Could you check a few things on this model? Use its own coordinates, in mm. A direction names the side the tool comes from. Give positions to 0.01 mm unless a question says otherwise; leave off trailing zeros. Write each loop counter-clockwise with the first axis right and the second up, starting at its lowest first coordinate (ties: lowest second). Pieces come first, ordered by that corner, then holes. Notation, with made-up numbers: M 28,-10 L 68,-10 A18 ccw 68,10 Z; hole C -29.75,55 d9. An arc over 180 degrees is marked long. One line per item, written item: value.
```python
from build123d import *

# Parameters (mm, degrees)
PAD_DEPTH            = 10
PAD002_DEPTH         = 29.635
POCKET_DEPTH         = 0.001
POCKET_DEPTH_BACK    = -14.001
SKETCH004_W          = 82.61631
SKETCH004_H          = 35.698411
SKETCH004_W_2        = 63.407177
SKETCH004_H_2        = 4.929781
POCKET001_DEPTH      = 17.005409
POCKET001_DEPTH_BACK = -17.005409


with BuildPart() as part:
    # Sketch → Pad (new body)
    with BuildSketch(Plane.XY):
        Polygon((19.635, 0), (9.8175, 17.004409), (-9.8175, 17.004409), (-19.635, 0), (-9.8175, -17.004409), (9.8175, -17.004409), align=None)
        Polygon((13.635, 0), (6.8175, 11.808256), (-6.8175, 11.808256), (-13.635, 0), (-6.8175, -11.808256), (6.8175, -11.808256), align=None, mode=Mode.SUBTRACT)
    extrude(amount=PAD_DEPTH)

    # Sketch002 → Pad002 (join, symmetric)
    with BuildSketch(Plane.YZ):
        with BuildLine():
            ThreePointArc((4, 10), (0, 14), (-4, 10))
            Line((-4, 10), (-4, 0))
            Line((-4, 0), (4, 0))
            Line((4, 0), (4, 10))
        make_face()
    extrude(amount=PAD002_DEPTH, both=True)

    # Sketch003 → Pocket (cut, two sides)
    with BuildSketch(Plane.XY) as pocket_sk:
        Polygon((13.635, 0), (6.8175, 11.808256), (-6.8175, 11.808256), (-13.635, 0), (-6.8175, -11.808256), (6.8175, -11.808256), align=None)
    extrude(amount=-POCKET_DEPTH, mode=Mode.SUBTRACT)
    extrude(pocket_sk.sketch, amount=-POCKET_DEPTH_BACK, mode=Mode.SUBTRACT)

    # Sketch004 → Pocket001 (cut, two sides)
    with BuildSketch(Plane.XZ) as pocket001_sk:
        with Locations((0.841957, 8.089457)):
            Rectangle(SKETCH004_W, SKETCH004_H)
        with Locations((0.246989, 0.581458)):
            Rectangle(SKETCH004_W_2, SKETCH004_H_2, mode=Mode.SUBTRACT)
    extrude(amount=-POCKET001_DEPTH, mode=Mode.SUBTRACT)
    extrude(pocket001_sk.sketch, amount=-POCKET001_DEPTH_BACK, mode=Mode.SUBTRACT)


solid = part.part
```
1) If we section it at A-A, the plane x = 1: Write out the boundary of the cut face in (y, z).
Outcome:
outline: M -17,0 L -11.81,0 L -11.81,3.05 L -17,3.05 Z; M 11.81,0 L 17,0 L 17,3.05 L 11.81,3.05 Z
2) We'd pull the mould along X, two halves only. Please class faces 1 (the face through (0, -17.004, 2)), 2 (the face through (-29.635, 0, 2)), 3 (the face through (13.624, 10.411, 1.502)), 4 (the face through (10.274, 5.821, 1.502)): pulls with the +X half, pulls with the -X half, needs draft (parallel to the pull), parting line crosses it, or undercut.
Outcome:
face 1: needs draft
face 2: pulls with the -X half
face 3: pulls with the +X half
face 4: undercut
3) On a 3-axis mill with a long thin cutter (end or side, diameter ignored), from which of +Z, -Z, +X, -X, +Y, -Y can I reach the whole of each face in a straight line? I mean faces 5 (the face through (-23, 4, 2)), 6 (the face through (24, 4, 2)), 7 (the face through (-23, -4, 2)), 8 (the face through (-10.274, -5.821, 1.502)), 9 (the face through (24, -4, 2)). Say none if no direction works.
Outcome:
face 5: +Z, -Z, -X, +Y
face 6: +Z, -Z, +X, +Y
face 7: +Z, -Z, -X, -Y
face 8: +Z, -Z
face 9: +Z, -Z, +X, -Y
4) If we section it at D-D, the plane x = 18: Write out the boundary of the cut face in (y, z).
Outcome:
outline: M -4,0 L 4,0 L 4,3.05 L -4,3.05 Z
5) I'm going to push flat-ended pins straight in: pin 1 (1.5 mm diameter, centred on x = -25, z = 1, fed in from -Y); pin 2 (1 mm diameter, centred on y = -5.5, z = 2.5, fed in from +X). Where does each tip first touch, or does it pass through?
Outcome:
pin 1: stops at y = -4
pin 2: stops at x = 16.75
6) Please list where these lines run through material, in increasing order: L1, parallel to Y at x = 3.5, z = 2.5; L2, parallel to X at y = 0, z = 0.8 (3 decimals); L3, parallel to Y at x = -19.5, z = 2.1. Write a range as from..to.
Outcome:
L1: y = -17..-11.81, 11.81..17
L2: x = -29.635..-13.635, 13.635..29.635
L3: y = -4..4
7) If we section it at C-C, the plane z = 2.4: Write out the boundary of the cut face in (x, y) (1 decimal), then the cut area to 3 significant figures.
Outcome:
outline: M -29.6,-4 L -17.3,-4 L -9.8,-17 L 9.8,-17 L 17.3,-4 L 29.6,-4 L 29.6,4 L 17.3,4 L 9.8,17 L -9.8,17 L -17.3,4 L -29.6,4 Z; hole M -13.6,0 L -6.8,-11.8 L 6.8,-11.8 L 13.6,0 L 6.8,11.8 L -6.8,11.8 Z
area: 697 mm^2
8) If we section it at B-B, the plane y = -9: Write out the boundary of the cut face in (x, z), then the cut area to 3 significant figures.
Outcome:
outline: M -14.44,0 L -8.44,0 L -8.44,3.05 L -14.44,3.05 Z; M 8.44,0 L 14.44,0 L 14.44,3.05 L 8.44,3.05 Z
area: 36.6 mm^2
